Source: three-view drawing plus pictorial views. Frame: mm from the lowest corner of the part. A direction names the side the tool comes from. Coordinates: 2 decimals unless noted, no trailing zeros. Write each loop counter-clockwise with the first axis right and the second up, starting at its lowest first coordinate (ties: lowest second). Pieces come first, ordered by that corner, then holes. Notation, with made-up numbers: M -0.75,38 L 45.25,38 A17 ccw 45.25,58 Z; hole C -10.5,7 d5. An arc over 180 degrees is marked long. Use CSV: the item, a comma, the result in double quotes.
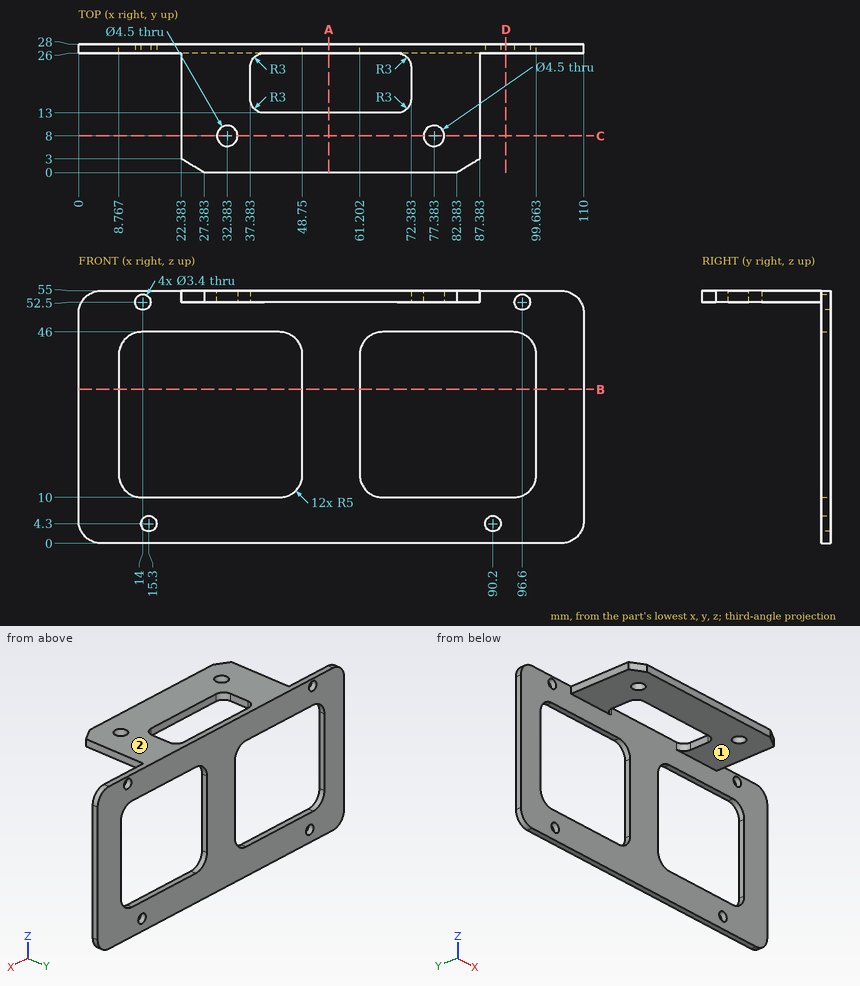
1. Section B-B (z = 33.5). Return loops of the section in (x, y).
Resolved:
outline,"M 0,26 L 8.77,26 L 8.77,28 L 0,28 Z; M 48.75,26 L 61.2,26 L 61.2,28 L 48.75,28 Z; M 99.66,26 L 110,26 L 110,28 L 99.66,28 Z"
2. Access query for the marked faces 1 and 2. Directions: +Z, -Z, +X, -X, +Y, -Y. A direction counts if a zero-diameter tool reaches every point of the face in a straight line with its end or side. Return the directions, or none.
Resolved:
face 1,"-Z, +X, -X, -Y"
face 2,"+Z, +X, -X, +Y, -Y"
3. Section C-C (y = 8). Return loops of the section in (x, z).
Resolved:
outline,"M 22.38,52.5 L 30.13,52.5 L 30.13,55 L 22.38,55 Z; M 34.63,52.5 L 75.13,52.5 L 75.13,55 L 34.63,55 Z; M 79.63,52.5 L 87.38,52.5 L 87.38,55 L 79.63,55 Z"
4. Section D-D (x = 93). Return loops of the section in (y, z).
Resolved:
outline,"M 26,0 L 28,0 L 28,10 L 26,10 Z; M 26,46 L 28,46 L 28,55 L 26,55 Z"
5. Section A-A (x = 54.5). Return loops of the section in (y, z).
Resolved:
outline,"M 0,52.5 L 13,52.5 L 13,55 L 0,55 Z; M 26,0 L 28,0 L 28,55 L 26,55 Z"
6. Contact query for flat-ended pins moving along their axis: pin 1 Ø0.8 at (y, z) = (19.5, 53.5) entering from +X; pin 2 Ø8 at (x, z) = (40.5, 7.5) entering from -Y; pin 3 Ø4 at (x, z) = (90.2, 4.3) entering from +Y; pin 4 Ø2 at (y, z) = (9, 54) entering from -X. Output: stop coordinate, or through.
Resolved:
pin 1,"stops at x = 87.38"
pin 2,"stops at y = 26"
pin 3,"stops at y = 28"
pin 4,"stops at x = 22.38"
7. Material intervals for line 1 (X direction, y = 27.65, z = 52.5); line 2 (X direction, y = 26.45, z = 4.3); line 3 (Z direction, x = 92, y = 26.5), sorted ascending. Write a range as [from, to].
Resolved:
line 1,"x = [0.67, 12.3], [15.7, 94.9], [98.3, 109.33]"
line 2,"x = [0.05, 13.6], [17, 88.5], [91.9, 109.95]"
line 3,"z = [0, 10], [46, 55]"
